Build history of the part. All positions in model axes, mm. Round coordinates to 2 decimals unless told otherwise and drop trailing zeros. Write each loop counter-clockwise with the first axis right and the second up, starting at its lowest first coordinate (ties: lowest second). Pieces come first, ordered by that corner, then holes. Notation, with made-up numbers: (9, -7.5) -> (45, -7.5) arc R25 ccw to (45, 12.5) -> close; hole circle Ø10 at (53.25, 41). An arc over 180 degrees is marked (long way). One line per question, with ' | ' between items.
from build123d import *

# Parameters (mm, degrees)
PAD015_DEPTH                        = 3
SKETCH054_R                         = 1.7
POCKET018_DEPTH                     = 0.001
POCKET018_DEPTH_BACK                = 3.001
BODY001003005003004_PLACEMENT_ANGLE = 60


with BuildPart() as part:
    # Sketch053 → Pad015 (new body)
    with BuildSketch(Plane.XY):
        with BuildLine():
            Line((0, 182.848457), (0, 197.848457))
            ThreePointArc((141.077868, 138.712102), (76.485413, 182.466418), (0, 197.848457))
            ThreePointArc((141.062279, 137.294387), (141.364747, 138.000004), (141.077868, 138.712102))
            Line((131.746186, 128.227134), (141.062279, 137.294387))
            ThreePointArc((130.335906, 128.242388), (131.037899, 127.943805), (131.746186, 128.227134))
            ThreePointArc((130.335906, 128.242388), (70.656336, 168.64531), (0, 182.848457))
        make_face()
    pad015 = extrude(amount=PAD015_DEPTH)

    # Mirrored020: Pad015 across Sketch053 V_Axis
    add(pad015.mirror(Plane(origin=(0, 0, 0), x_dir=(0, 0, 1), z_dir=(1, 0, 0))))

    # Sketch054 → Pocket018 (cut, two sides)
    with BuildSketch(Plane.XY) as pocket018_sk:
        with Locations((129.243686, 139.741203)):
            Circle(SKETCH054_R)
        with Locations((0, 190.345828)):
            Circle(SKETCH054_R)
        with Locations((-129.243686, 139.741203)):
            Circle(SKETCH054_R)
    extrude(amount=-POCKET018_DEPTH, mode=Mode.SUBTRACT)
    extrude(pocket018_sk.sketch, amount=POCKET018_DEPTH_BACK, mode=Mode.SUBTRACT)


with BuildPart() as part_1:
    # Body001003005003004 placement: moved
    add(part.part.rotate(Axis((0, 0, 0), (0, 0, 1)), BODY001003005003004_PLACEMENT_ANGLE))


solid = part_1.part
(1) Slice it at C-C (y = -18.5). Write the cut outline in (x, z), then the cut area to 3 significant figures.
Calculated:
outline: (-196.98, 0) -> (-181.91, 0) -> (-181.91, 3) -> (-196.98, 3) -> close | area: 45.2 mm2
(2) Wall check: line 1 (Y direction, x = -148, z = 1.95); line 2 (X direction, y = 26, z = 1); line 3 (X direction, y = -4.5, z = 2.85). Give the ranges that are in metal, low to high. Write a range as from..to.
Calculated:
line 1: 107.38..131.3 | line 2: -196.13..-180.99 | line 3: -197.8..-182.79
(3) Slice it at A-A (z = 2.3). Write the cut outline in (x, y), then the cut area to 3 significant figures.
Calculated:
outline: (-190.67, -52.82) arc R1 ccw to (-189.43, -53.52) -> (-176.92, -49.98) arc R1 ccw to (-176.23, -48.75) arc R182.85 cw to (-158.35, 91.42) arc R182.85 cw to (-45.89, 177) arc R1 ccw to (-45.17, 178.21) -> (-48.37, 190.81) arc R1 ccw to (-49.59, 191.53) arc R197.85 ccw to (-171.34, 98.92) arc R197.85 ccw to start; hole circle Ø3.4 at (-185.64, -42.06); hole circle Ø3.4 at (-164.84, 95.17); hole circle Ø3.4 at (-56.4, 181.8) | area: 4,530 mm2
(4) Slice it at B-B (x = -121.5). Write the cut outline in (y, z), then the cut area to 3 significant figures.
Calculated:
outline: (136.64, 0) -> (156.15, 0) -> (156.15, 3) -> (136.64, 3) -> close | area: 58.5 mm2
(5) Drop flat-ended pins along their axis: pin 1 (1.5 mm diameter, centred on x = -126, z = 1, fed in from +Y) (3 decimals); pin 2 (1 mm diameter, centred on x = -104, z = 0.5, fed in from +Y). Give the stop position or say it passes through.
Calculated:
pin 1: y = 153.155 | pin 2: y = 168.62
